from build123d import *

# Parameters (mm, degrees)
SKETCH003_W     = 15.5
SKETCH003_H     = 21
PAD002_DEPTH    = 1.2
CHAMFER_SIZE    = 0.75
SKETCH004_R     = 1.65
POCKET001_DEPTH = 5


with BuildPart() as part:
    # Sketch003 → Pad002 (new body)
    with BuildSketch(Plane.XY):
        with Locations((-0.75, 0)):
            Rectangle(SKETCH003_W, SKETCH003_H)
    extrude(amount=PAD002_DEPTH)

    # Chamfer
    chamfer_edges = [part.edges().sort_by_distance(p)[0] for p in [
        (-8.5, -10.5, 0.6),
        (7, 10.5, 0.6),
        (7, -10.5, 0.6),
        (-8.5, 10.5, 0.6),
    ]]
    chamfer(chamfer_edges, length=CHAMFER_SIZE)

    # Sketch004 (on Face5 of Chamfer) → Pocket001 (cut)
    with BuildSketch(Plane.XY.offset(1.2)):
        with Locations((4.275, 7.775)):
            Circle(SKETCH004_R)
        with Locations((4.275, -7.775)):
            Circle(SKETCH004_R)
    extrude(amount=-POCKET001_DEPTH, mode=Mode.SUBTRACT)


with BuildPart() as part_1:
    # Body placement: moved
    add(part.part.moved(Location((0, 0, -1.65))))


solid = part_1.part
Check sheet for the modelled part. Datum: model origin and axes. Units: mm. Round coordinates to 2 decimals unless told otherwise and drop trailing zeros. Order: outer loops, then holes, each group sorted by start corner. A loop starts at its lowest first (then second) coordinate and runs counter-clockwise, first axis right, second up.
(1) Cross-section at B-B, the plane y = -9. Enter the section's corners in (x, z), and give its area (3 significant figures).
(2) Cross-section at A-A, the plane x = 3.5. Enter the section's corners in (y, z).
(3) Scan lines: probe 1 along Y at (x, z) = (3.25, -1.15); probe 2 along X at (y, z) = (7.75, -0.5); probe 3 along Y at (x, z) = (5.75, -1.15). Record each from-to range of solid material in increasing order.
(4) Cross-section at C-C, the plane z = -1. Enter the section's corners in (x, y) (3 decimals).
Check sheet entries:
1. outline: (-8.5, -1.65) - (3.17, -1.65) - (3.17, -0.45) - (-8.5, -0.45) - close; (5.38, -1.65) - (7, -1.65) - (7, -0.45) - (5.38, -0.45) - close
1. area: 15.9 mm2
2. outline: (-10.5, -1.65) - (-9.23, -1.65) - (-9.23, -0.45) - (-10.5, -0.45) - close; (-6.32, -1.65) - (6.32, -1.65) - (6.32, -0.45) - (-6.32, -0.45) - close; (9.23, -1.65) - (10.5, -1.65) - (10.5, -0.45) - (9.23, -0.45) - close
3. probe 1: y = -10.5 to -9.07, -6.48 to 6.48, 9.07 to 10.5
3. probe 2: x = -8.5 to 2.63, 5.92 to 7
3. probe 3: y = -10.5 to -8.51, -7.04 to 7.04, 8.51 to 10.5
4. outline: (-8.5, -9.75) - (-7.75, -10.5) - (6.25, -10.5) - (7, -9.75) - (7, 9.75) - (6.25, 10.5) - (-7.75, 10.5) - (-8.5, 9.75) - close; hole circle Ø3.3 at (4.275, -7.775); hole circle Ø3.3 at (4.275, 7.775)
